Source: CAD feature listing. Evaluate the final solid. Frame: model axes, mm. A direction names the side the tool comes from. Round coordinates to 2 decimals unless told otherwise and drop trailing zeros. Write each loop counter-clockwise with the first axis right and the second up, starting at its lowest first coordinate (ties: lowest second). Pieces come first, ordered by that corner, then holes. Notation, with made-up numbers: M -38.75,37 L 15.25,37 A20 cw 15.25,44 Z; hole C 36,72 d3. An arc over 180 degrees is marked long. Use a Markdown table: item, result.
```python
from build123d import *

# Parameters (mm, degrees)
CYLINDER078_R     = 0.8
CYLINDER078_DEPTH = 14.5
CYLINDER077_R     = 0.8
CYLINDER077_DEPTH = 14.5
BOX042_W          = 5.3
BOX042_H          = 8
BOX042_DEPTH      = 10
BOX041_W          = 14
BOX041_H          = 6
BOX041_DEPTH      = 10
BOX040_W          = 30
BOX040_H          = 15
BOX040_DEPTH      = 1.6


with BuildPart() as cylinder130:
    # Cylinder078 → Cylinder078 (new body)
    with BuildSketch(Plane(origin=(-43.6, -13.8, -9), x_dir=(1, 0, 0), z_dir=(0, 0, 1))):
        Circle(CYLINDER078_R)
    extrude(amount=CYLINDER078_DEPTH)


with BuildPart() as fusion109:
    # Cylinder077 → Cylinder077 (new body)
    with BuildSketch(Plane(origin=(-43.6, -2.4, -9), x_dir=(1, 0, 0), z_dir=(0, 0, 1))):
        Circle(CYLINDER077_R)
    extrude(amount=CYLINDER077_DEPTH)

    # Fusion109: union Cylinder130
    add(cylinder130.part)


with BuildPart() as cube040:
    # Box042 → Box042 (new body)
    with BuildSketch(Plane(origin=(-51.7, -11.5, -4.5), x_dir=(1, 0, 0), z_dir=(0, 0, 1))):
        with Locations((2.65, 4)):
            Rectangle(BOX042_W, BOX042_H)
    extrude(amount=BOX042_DEPTH)


with BuildPart() as cut045025:
    # Box041 → Box041 (new body)
    with BuildSketch(Plane(origin=(-56, -10.5, -4.5), x_dir=(1, 0, 0), z_dir=(0, 0, 1))):
        with Locations((7, 3)):
            Rectangle(BOX041_W, BOX041_H)
    extrude(amount=BOX041_DEPTH)

    # Cut045025: cut Cube040
    add(cube040.part, mode=Mode.SUBTRACT)


with BuildPart() as spoke_sensor_pcb001:
    # Box040 → Box040 (new body)
    with BuildSketch(Plane(origin=(-56, -15.5, -6), x_dir=(1, 0, 0), z_dir=(0, 0, 1))):
        with Locations((15, 7.5)):
            Rectangle(BOX040_W, BOX040_H)
    extrude(amount=BOX040_DEPTH)

    # Fusion108: union Cut045025
    add(cut045025.part)

    # Cut045026: cut Fusion109
    add(fusion109.part, mode=Mode.SUBTRACT)


solid = spoke_sensor_pcb001.part
```
Q1. Section B-B on x = -43.6. Return loops of the section in (y, z).
Results are:
| item | result |
|---|---|
| outline | M -15.5,-6 L -14.6,-6 L -14.6,-4.4 L -15.5,-4.4 Z; M -13,-6 L -3.2,-6 L -3.2,-4.4 L -4.5,-4.4 L -4.5,5.5 L -10.5,5.5 L -10.5,-4.4 L -13,-4.4 Z; M -1.6,-6 L -0.5,-6 L -0.5,-4.4 L -1.6,-4.4 Z |
Q2. Reachability of faces 1 (the flat face through (-51.7, -8, 0)), 2 (the flat face through (-54, -10.5, 0)), 3 (the flat face through (-42, -8, 0)) from +Z, -Z, +X, -X, +Y, -Y: full face, straight path, thin tool, end or side. Return the list, or none.
Results are:
| item | result |
|---|---|
| face 1 | +Z, +Y, -Y |
| face 2 | +Z, +X, -X, -Y |
| face 3 | +Z, +X, +Y, -Y |
Q3. Line query: L1, parallel to Y at x = -43.6, z = -4.95; L2, parallel to X at y = -2.4, z = -4.8; L3, parallel to X at y = -8.5, z = -3. Output: solid intervals per line, ascending.
Results are:
| item | result |
|---|---|
| L1 | -15.5 to -14.6, -13 to -3.2, -1.6 to -0.5 |
| L2 | -56 to -44.4, -42.8 to -26 |
| L3 | -56 to -51.7, -46.4 to -42 |
Q4. Section C-C on y = -13.8. Return loops of the section in (x, z), plus the area to 3 significant figures.
Results are:
| item | result |
|---|---|
| outline | M -56,-6 L -44.4,-6 L -44.4,-4.4 L -56,-4.4 Z; M -42.8,-6 L -26,-6 L -26,-4.4 L -42.8,-4.4 Z |
| area | 45.4 mm^2 |
Q5. Mould query, pull axis Y, two halves, no side actions, for faces 4 (the flat face through (-41, -8, -4.4)), 5 (the flat face through (-54, -4.5, 0)), 6 (the cylindrical face through (-42.861, -14.106, -5.211)), 7 (the cylindrical face through (-42.861, -2.706, -5.211)). Classes: +Y half, -Y half, draft (parallel to the pull), parting line (faces both ways), or undercut.
Results are:
| item | result |
|---|---|
| face 4 | draft |
| face 5 | +Y half |
| face 6 | undercut |
| face 7 | undercut |
Q6. Section A-A on z = -3. Return loops of the section in (x, y).
Results are:
| item | result |
|---|---|
| outline | M -56,-10.5 L -51.7,-10.5 L -51.7,-4.5 L -56,-4.5 Z; M -46.4,-10.5 L -42,-10.5 L -42,-4.5 L -46.4,-4.5 Z |
Q7. First-contact query: pin 1 Ø2 at (x, z) = (-44.5, 1.5) entering from -Y; pin 2 Ø3.5 at (x, z) = (-54, -1) entering from +Y; pin 3 Ø1.5 at (y, z) = (-12.5, 2.5) entering from -X; pin 4 Ø1.8 at (y, z) = (-6.5, 0) entering from +X. Flat tips, straight axial feed; report the tip coordinate or a pass-through.
Results are:
| item | result |
|---|---|
| pin 1 | y = -10.5 |
| pin 2 | y = -4.5 |
| pin 3 | through |
| pin 4 | x = -42 |
Q8. Section D-D on x = -54. Return loops of the section in (y, z), plus the area to 3 significant figures.
Results are:
| item | result |
|---|---|
| outline | M -15.5,-6 L -0.5,-6 L -0.5,-4.4 L -4.5,-4.4 L -4.5,5.5 L -10.5,5.5 L -10.5,-4.4 L -15.5,-4.4 Z |
| area | 83.4 mm^2 |
